The listing builds one solid part. Answer for the finished solid, in the listing's coordinates (mm). Face numbers are marked on the shaded views. A direction names the side the tool comes from. Give positions to 0.01 mm unless a question says otherwise; leave off trailing zeros. Order: outer loops, then holes, each group sorted by start corner. A loop starts at its lowest first (then second) coordinate and runs counter-clockwise, first axis right, second up. Notation, with made-up numbers: (22.5, 37.5) - (26.5, 37.5) arc R6 ccw to (26.5, 44.5) - close; hole circle Ø4 at (30, 81.5). An arc over 180 degrees is marked (long way). Answer as a JSON object with one key per item and string values. Group by question number.
Q1. Consider line 1 (Y direction, x = 18.05, z = 0.3); line 2 (X direction, y = -4, z = 10.5); line 3 (Z direction, x = 8, y = 0.5). Determine where each line is inside the solid, lowest interval first.
Q2. A cutting plane is placed at D-D, the plane z = 11.5. Give the vertices of the cut face in (x, y).
Q3. A cutting plane is placed at A-A, the plane x = -5.95. Give the vertices of the cut face in (y, z).
Q4. For the marked faces 1 and 2, determine the directions among +Z, -Z, +X, -X, +Y, -Y from which every point of the face is accessible in a straight line to the end or side of a thin tool.
Q5. A cutting plane is placed at C-C, the plane y = 4.75. Give the vertices of the cut face in (x, z), and give its area (3 significant figures).
Q6. Given pin 1 (2 mm diameter, centred on x = -5, y = -3.5, fed in from +Z); pin 2 (4.5 mm diameter, centred on y = -1, z = 19.5, fed in from +X), each flat-ended and moving along its own axis, determine where each tip first touches the part or whether it passes through.
Q7. A cutting plane is placed at B-B, the plane z = 19.8. Give the vertices of the cut face in (x, y), and give its area (3 significant figures).
from build123d import *

# Parameters (mm, degrees)
SKETCH_W        = 51.5
SKETCH_H        = 15
PAD_DEPTH       = 2
SKETCH001_W     = 2
SKETCH001_H     = 15
PAD001_DEPTH    = 49.5
FILLET_R        = 1.5
FILLET001_R     = 1
SKETCH002_R     = 2.2
POCKET_DEPTH    = 2.001
FILLET002_R     = 0.7
SKETCH003_R     = 2.2
POCKET001_DEPTH = 2.001
FILLET003_R     = 0.7


with BuildPart() as part:
    # Sketch → Pad (new body)
    with BuildSketch(Plane.XY):
        Rectangle(SKETCH_W, SKETCH_H)
    extrude(amount=PAD_DEPTH)

    # Sketch001 (on Face6 of Pad) → Pad001 (join)
    with BuildSketch(Plane.XY.offset(2)):
        with Locations((-24.75, 0)):
            Rectangle(SKETCH001_W, SKETCH001_H)
    extrude(amount=PAD001_DEPTH)

    # Fillet
    fillet_edges = [part.edges().sort_by_distance(p)[0] for p in [
        (-25.75, 0, 0),
    ]]
    fillet(fillet_edges, radius=FILLET_R)

    # Fillet001
    fillet001_edges = [part.edges().sort_by_distance(p)[0] for p in [
        (-23.75, 0, 2),
    ]]
    fillet(fillet001_edges, radius=FILLET001_R)

    # Sketch002 (on Face2 of Fillet001) → Pocket (cut, through all)
    with BuildSketch(Plane.XY.offset(2)):
        with Locations((18.05, 0)):
            Circle(SKETCH002_R)
        with Locations((-5.95, 0)):
            Circle(SKETCH002_R)
    extrude(amount=-POCKET_DEPTH, mode=Mode.SUBTRACT)

    # Fillet002
    fillet002_edges = [part.edges().sort_by_distance(p)[0] for p in [
        (15.85, 0, 2),
        (-8.15, 0, 2),
    ]]
    fillet(fillet002_edges, radius=FILLET002_R)

    # Sketch003 (on Face14 of Fillet002) → Pocket001 (cut, through all)
    with BuildSketch(Plane.YZ.offset(-23.75)):
        with Locations((0, 43.8)):
            Circle(SKETCH003_R)
        with Locations((0.10123, 19.8)):
            Circle(SKETCH003_R)
    extrude(amount=-POCKET001_DEPTH, mode=Mode.SUBTRACT)

    # Fillet003
    fillet003_edges = [part.edges().sort_by_distance(p)[0] for p in [
        (-23.75, -2.2, 43.8),
        (-23.75, -2.09877, 19.8),
    ]]
    fillet(fillet003_edges, radius=FILLET003_R)


solid = part.part
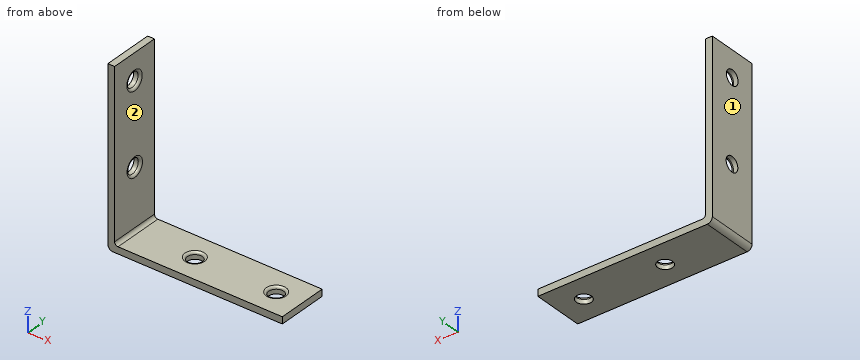
Reply:
{
 "1": {"line 1": "y = -7.5 to -2.2, 2.2 to 7.5", "line 2": "x = -25.75 to -23.75", "line 3": "z = 0 to 2"},
 "2": {"outline": "(-25.75, -7.5) - (-23.75, -7.5) - (-23.75, 7.5) - (-25.75, 7.5) - close"},
 "3": {"outline": "(-7.5, 0) - (-2.2, 0) - (-2.2, 1.3) arc R0.7 ccw to (-2.9, 2) - (-7.5, 2) - close; (2.2, 0) - (7.5, 0) - (7.5, 2) - (2.9, 2) arc R0.7 ccw to (2.2, 1.3) - close"},
 "4": {"face 1": "+Z, -Z, -X, +Y, -Y", "face 2": "+Z, +X, +Y, -Y"},
 "5": {"outline": "(-25.75, 1.5) arc R1.5 ccw to (-24.25, 0) - (25.75, 0) - (25.75, 2) - (-22.75, 2) arc R1 cw to (-23.75, 3) - (-23.75, 51.5) - (-25.75, 51.5) - close", "area": "202 mm^2"},
 "6": {"pin 1": "stops at z = 2", "pin 2": "stops at x = -23.75"},
 "7": {"outline": "(-25.75, -7.5) - (-23.75, -7.5) - (-23.75, -2.8) arc R0.7 ccw to (-24.45, -2.1) - (-25.75, -2.1) - close; (-25.75, 2.3) - (-24.45, 2.3) arc R0.7 ccw to (-23.75, 3) - (-23.75, 7.5) - (-25.75, 7.5) - close", "area": "21.0 mm^2"}
}
